from build123d import *

# Parameters (mm, degrees)
SKETCH1_W            = 25.5
SKETCH1_H            = 14
BOSS_EXTRUDE1_DEPTH  = 4
SKETCH2_R            = 1.5
CUT_EXTRUDE1_DEPTH   = 53.71750714
SKETCH3_W            = 30.5
SKETCH3_H            = 4
BOSS_EXTRUDE2_DEPTH  = 5.1
SKETCH4_W            = 30.5
SKETCH4_H            = 3
BOSS_EXTRUDE3_DEPTH  = 21
SKETCH5_W            = 30.5
SKETCH5_H            = 2
BOSS_EXTRUDE8_DEPTH  = 14.8
SKETCH10_W           = 30.5
SKETCH10_H           = 2
BOSS_EXTRUDE9_DEPTH  = 16.8
SKETCH11_W           = 1.5
SKETCH11_H           = 12.8
BOSS_EXTRUDE10_DEPTH = 4.6
SKETCH13_W           = 15.25
SKETCH13_H           = 2
BOSS_EXTRUDE11_DEPTH = 15.75
SKETCH14_W           = 10
SKETCH14_H           = 5
CUT_EXTRUDE5_DEPTH   = 3
SKETCH16_R           = 1
CUT_EXTRUDE6_DEPTH   = 10
SKETCH15_W           = 14.75
SKETCH15_H           = 3
BOSS_EXTRUDE12_DEPTH = 9.55
SKETCH18_W           = 30.5
SKETCH18_H           = 4
BOSS_EXTRUDE13_DEPTH = 32
SKETCH19_W           = 30.5
SKETCH19_H           = 3
BOSS_EXTRUDE14_DEPTH = 2.1
BOSS_EXTRUDE17_DEPTH = 4
SKETCH24_W           = 3.969230492
SKETCH24_H           = 32
BOSS_EXTRUDE18_DEPTH = 66.85


with BuildPart() as part:
    # Sketch1 → Boss-Extrude1 (new body)
    with BuildSketch(Plane(origin=(0, 0, 0), x_dir=(1, 0, 0), z_dir=(0, 1, 0))):
        Polygon((-36.234375, 16.8984375), (-41.234375, 16.8984375), (-41.234375, -32.6015625), (-36.234375, -32.6015625), (-36.234375, 2.8984375), align=None)
        with Locations((-23.484375, 9.8984375)):
            Rectangle(SKETCH1_W, SKETCH1_H)
    extrude(amount=BOSS_EXTRUDE1_DEPTH)

    # Sketch2 → Cut-Extrude1 (cut, through all)
    with BuildSketch(Plane(origin=(0, 4, 0), x_dir=(1, 0, 0), z_dir=(0, 1, 0))):
        with Locations(Location((-38.984375, -29.3515625, 0), (0, 0, 270))):
            Circle(SKETCH2_R)
        with Locations(Location((-38.984375, 12.6484375, 0), (0, 0, 270))):
            Circle(SKETCH2_R)
        with Locations(Location((-13.984375, 12.6484375, 0), (0, 0, 270))):
            Circle(SKETCH2_R)
    extrude(amount=-CUT_EXTRUDE1_DEPTH, mode=Mode.SUBTRACT)

    # Sketch3 → Boss-Extrude2 (add)
    with BuildSketch(Plane(origin=(0, 0, -16.8984375), x_dir=(-1, 0, 0), z_dir=(0, 0, -1))):
        with Locations((25.984375, 2)):
            Rectangle(SKETCH3_W, SKETCH3_H)
    extrude(amount=BOSS_EXTRUDE2_DEPTH)

    # Sketch4 → Boss-Extrude3 (add)
    with BuildSketch(Plane.XZ):
        with Locations((-25.984375, -20.4984375)):
            Rectangle(SKETCH4_W, SKETCH4_H)
    extrude(amount=BOSS_EXTRUDE3_DEPTH)

    # Sketch5 → Boss-Extrude8 (add)
    with BuildSketch(Plane(origin=(0, 0, -21.9984375), x_dir=(-1, 0, 0), z_dir=(0, 0, -1))):
        with Locations((25.984375, -20)):
            Rectangle(SKETCH5_W, SKETCH5_H)
    extrude(amount=BOSS_EXTRUDE8_DEPTH)

    # Sketch10 → Boss-Extrude9 (add)
    with BuildSketch(Plane(origin=(0, -19, 0), x_dir=(1, 0, 0), z_dir=(0, 1, 0))):
        with Locations((-25.984375, 35.7984375)):
            Rectangle(SKETCH10_W, SKETCH10_H)
    extrude(amount=BOSS_EXTRUDE9_DEPTH)

    # Sketch11 → Boss-Extrude10 (add)
    with BuildSketch(Plane(origin=(0, -19, 0), x_dir=(1, 0, 0), z_dir=(0, 1, 0))):
        with Locations((-11.484375, 28.3984375)):
            Rectangle(SKETCH11_W, SKETCH11_H)
    boss_extrude10 = extrude(amount=BOSS_EXTRUDE10_DEPTH)

    # Sketch13 → Boss-Extrude11 (add)
    with BuildSketch(Plane(origin=(0, -2.2, 0), x_dir=(1, 0, 0), z_dir=(0, 1, 0))):
        with Locations((-18.359375, 35.7984375)):
            Rectangle(SKETCH13_W, SKETCH13_H)
    extrude(amount=BOSS_EXTRUDE11_DEPTH)

    # Sketch14 → Cut-Extrude5 (cut)
    with BuildSketch(Plane.XY.offset(-18.9984375)):
        with Locations((-30.706752917, -15.5)):
            Rectangle(SKETCH14_W, SKETCH14_H)
    extrude(amount=-CUT_EXTRUDE5_DEPTH, mode=Mode.SUBTRACT)

    # Sketch16 → Cut-Extrude6 (cut)
    with BuildSketch(Plane(origin=(-10.734375, 0, 0), x_dir=(0, 0, -1), z_dir=(1, 0, 0))):
        with Locations((30.286455297, -15.059839978)):
            Circle(SKETCH16_R)
    cut_extrude6 = extrude(amount=-CUT_EXTRUDE6_DEPTH, mode=Mode.SUBTRACT)

    # Mirror1: Boss-Extrude10, Cut-Extrude6 across plane
    add(boss_extrude10.mirror(Plane(origin=(0, -2.725, 0), x_dir=(0, 0, 1), z_dir=(0, -1, 0))))
    add(cut_extrude6.mirror(Plane(origin=(0, -2.725, 0), x_dir=(0, 0, 1), z_dir=(0, -1, 0))), mode=Mode.SUBTRACT)

    # Sketch15 → Boss-Extrude12 (add)
    with BuildSketch(Plane(origin=(0, 4, 0), x_dir=(1, 0, 0), z_dir=(0, 1, 0))):
        with Locations((-18.109375, 20.4984375)):
            Rectangle(SKETCH15_W, SKETCH15_H)
    extrude(amount=BOSS_EXTRUDE12_DEPTH)

    # Sketch18 → Boss-Extrude13 (add)
    with BuildSketch(Plane.XZ.offset(21)):
        with Locations((-25.984375, -20.9984375)):
            Rectangle(SKETCH18_W, SKETCH18_H)
    extrude(amount=BOSS_EXTRUDE13_DEPTH)

    # Sketch19 → Boss-Extrude14 (add)
    with BuildSketch(Plane.XY.offset(-18.9984375)):
        with Locations((-25.984375, -51.5)):
            Rectangle(SKETCH19_W, SKETCH19_H)
    extrude(amount=BOSS_EXTRUDE14_DEPTH)

    # Sketch20 → Boss-Extrude17 (add)
    with BuildSketch(Plane(origin=(0, 0, -22.9984375), x_dir=(-1, 0, 0), z_dir=(0, 0, -1))):
        Polygon((14.734375, -24.112056249), (14.734375, -23), (17.020268401, -23), (41.234375, -23), (41.234375, -21), (10.734375, -21), (10.734375, -53), (41.234375, -53), (41.234375, -50), (17.020268401, -50), (14.734375, -50), (14.734375, -48.887943751), align=None)
        Polygon((41.234375, -21), (41.234375, -23), (67.948481599, -23), (70.234375, -23), (70.234375, -24.112056249), (70.234375, -48.887943751), (70.234375, -50), (67.948481599, -50), (41.234375, -50), (41.234375, -53), (74.234375, -53), (74.234375, -21), align=None)
        Polygon((17.020268401, -23), (14.734375, -23), (14.734375, -24.112056249), (40.198481599, -36.5), (14.734375, -48.887943751), (14.734375, -50), (17.020268401, -50), (41.234375, -38.220164357), (41.234375, -34.779835643), align=None)
        Polygon((42.484375, -35.387943751), (41.234375, -34.779835643), (41.234375, -38.220164357), (42.484375, -37.612056249), (67.948481599, -50), (70.234375, -50), (70.234375, -48.887943751), (44.770268401, -36.5), (70.234375, -24.112056249), (70.234375, -23), (67.948481599, -23), align=None)
    extrude(amount=BOSS_EXTRUDE17_DEPTH)

    # Sketch24 → Boss-Extrude18 (add)
    with BuildSketch(Plane(origin=(0, 0, -26.9984375), x_dir=(-1, 0, 0), z_dir=(0, 0, -1))):
        with Locations((72.249759754, -37)):
            Rectangle(SKETCH24_W, SKETCH24_H)
    extrude(amount=BOSS_EXTRUDE18_DEPTH)


solid = part.part
Could you check a few things on this model? Use its own coordinates, in mm. A direction names the side the tool comes from. Coordinates: 2 decimals unless noted, no trailing zeros. Order: outer loops, then holes, each group sorted by start corner. A loop starts at its lowest first (then second) coordinate and runs counter-clockwise, first axis right, second up. Notation, with made-up numbers: (41, 88.25) -> (72, 88.25) arc R18 cw to (72, 105.25) -> close; hole circle Ø6 at (46, 52.25). An arc over 180 degrees is marked (long way). One line per item, written item: value. Start each with the question number.
1) Imagine slicing it at D-D on y = -46. Count the separate pieces of the cut face and the enclosed holes in it, plus the area to 3 significant figures.
2) We'd pull the mould along Y, two halves only. Please class faces 6 (the flat face through (-43, -50, -25)), 7 (the flat face through (-12.234, 11, -28)), 8 (the flat face through (-71, -21, -45)): +Y half, -Y half, draft (parallel to the pull), parting line (faces both ways), or undercut.
3) Imagine slicing it at A-A on z = -33. List the corners of the cut face in (x, y) for me, plus the area to 3 significant figures.
4) Imagine slicing it at B-B on y = 7. List the corners of the cut face in (x, z) for me.
5) I'm going to push flat-ended pins straight in: pin 1 (5 mm diameter, centred on x = -37, z = 14.5, fed in from +Y); pin 2 (5 mm diameter, centred on y = 11.5, z = -27, fed in from -X); pin 3 (2 mm diameter, centred on y = 4.5, z = -35.5, fed in from -X). Where does each tip first touch, or does it pass through?
6) If I drill on L1, parallel to Z at x = -17.5, y = -8; L2, parallel to X at y = 10.5, z = -27; L3, parallel to Y at x = -39.5, z = -10, over which ranges is the centre line in solid material (lowest first)? Write a range as [from, to].
7) Which directions (+Z, -Z, +X, -X, +Y, -Y) give clear straight access to the entire face, cutting with the end or side of a thin tool? Please do faces 1 (the flat face through (-33.5, -40.3, -26.998)), 2 (the flat face through (-55, -43.7, -25)), 3 (the flat face through (-36.234, 2, 15)), 4 (the flat face through (-31, -13, -20)), 5 (the flat face through (-14.734, -37, -25)).
Answer list:
1. separate pieces: 3
1. enclosed holes: 0
1. area: 456 mm2
2. face 6: undercut
2. face 7: draft
2. face 8: +Y half
3. outline: (-74.23, -53) -> (-70.27, -53) -> (-70.27, -21) -> (-74.23, -21) -> close; (-41.23, -21) -> (-10.73, -21) -> (-10.73, -14.4) -> (-12.23, -14.4) -> (-12.23, -19) -> (-41.23, -19) -> close; (-12.23, 8.95) -> (-10.73, 8.95) -> (-10.73, 13.55) -> (-12.23, 13.55) -> close
3. area: 202 mm2
4. outline: (-25.98, -36.8) -> (-10.73, -36.8) -> (-10.73, -34.8) -> (-25.98, -34.8) -> close; (-25.48, -22) -> (-10.73, -22) -> (-10.73, -19) -> (-25.48, -19) -> close
5. pin 1: stops at y = 4
5. pin 2: stops at x = -12.23
5. pin 3: stops at x = -25.98
6. L1: z = [-36.8, -34.8], [-22, -19]
6. L2: x = [-12.23, -10.73]
6. L3: y = [0, 4]
7. face 1: -Z, +X, -Y
7. face 2: +Z, -Z
7. face 3: +Z, +X, +Y, -Y
7. face 4: +Z
7. face 5: -Z
